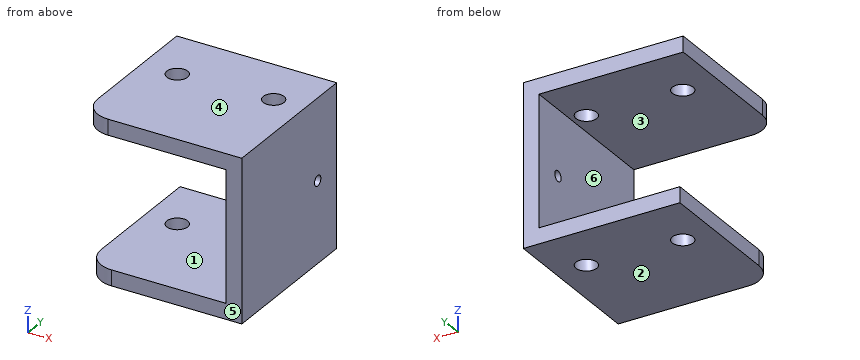
```python
from build123d import *

# Parameters (mm, degrees)
F1_DEPTH = 30
F3_D     = 2
F5_D     = 4
F6_R     = 5
F7_R     = 5


with BuildPart() as f1:
    # F0 (on Front) → F1 (new body)
    with BuildSketch(Plane.XZ):
        Polygon((-25.762998, -16.926608), (-25.762998, -19.926608), (4.237002, -19.926608), (4.237002, 11.073392), (-26.395301, 11.073392), (-26.395301, 8.073392), (1.237002, 8.073392), (1.237002, -16.926608), align=None)
    extrude(amount=F1_DEPTH)

    # F3 (through all)
    with Locations(Plane.YZ.offset(4.237002)):
        with Locations((-6, -4.426608)):
            Hole(F3_D / 2)

    # F5 (through all)
    with Locations(Plane(origin=(0, 0, -19.926608), x_dir=(1, 0, 0), z_dir=(0, 0, -1))):
        with Locations((-19.609278, 11.052052), (-1.659339, 10.208893)):
            Hole(F5_D / 2)

    # F6
    f6_edges = [f1.edges().sort_by_distance(p)[0] for p in [
        (-26.395301, -30, 9.573392),
    ]]
    fillet(f6_edges, radius=F6_R)

    # F7
    f7_edges = [f1.edges().sort_by_distance(p)[0] for p in [
        (-25.762998, -30, -18.426608),
    ]]
    fillet(f7_edges, radius=F7_R)


solid = f1.part
```
Verification items for the finished model (mm, model axes). Face numbers are marked on the shaded views. A direction names the side the tool comes from. Coordinates: 2 decimals unless noted, no trailing zeros. Loops run counter-clockwise (first coordinate to the right, second up) from the corner with the lowest first, then second, coordinate; pieces in that order, holes last. Notation, with made-up numbers: (32, 63) - (84, 63) arc R33 cw to (84, 100) - close; hole circle Ø2 at (48, 71.25). An arc over 180 degrees is marked (long way). Answer as a JSON object with one key per item and string values.
(1) Scan lines: line 1 along Z through (x, y) = (-9, -12); line 2 along Z through (x, y) = (3.15, -6); line 3 along X through (y, z) = (-24.5, 3). Record each from-to range of solid material in increasing order.
Response:
{"line 1": "z = -19.93 to -16.93, 8.07 to 11.07", "line 2": "z = -19.93 to -5.43, -3.43 to 11.07", "line 3": "x = 1.24 to 4.24"}
(2) Mould release check, pull along Z, two halves, no side actions. Record for the marked faces 3, 4, 5 and 6: pulls with the +Z half, pulls with the -Z half, needs draft (parallel to the pull), parting line crosses it, or undercut.
Response:
{"face 3": "undercut", "face 4": "pulls with the +Z half", "face 5": "needs draft", "face 6": "undercut"}
(3) Go/stop test with flat-tipped pins: pin 1 Ø3 at (x, y) = (-1.66, -10.21) entering from +Z; pin 2 Ø2.5 at (y, z) = (-7.5, -19) entering from -X; pin 3 Ø7.5 at (y, z) = (-9, -7.5) entering from -X. Record where each tip stops, or that it passes through.
Response:
{"pin 1": "passes through", "pin 2": "stops at x = -25.76", "pin 3": "stops at x = 1.24"}
(4) Cross-section at B-B, the plane y = -6. Record the boundary of the cut face in (x, z).
Response:
{"outline": "(-26.4, 8.07) - (1.24, 8.07) - (1.24, -3.43) - (4.24, -3.43) - (4.24, 11.07) - (-26.4, 11.07) - close; (-25.76, -19.93) - (4.24, -19.93) - (4.24, -5.43) - (1.24, -5.43) - (1.24, -16.93) - (-25.76, -16.93) - close"}
(5) Cross-section at A-A, the plane x = -4.5. Record the boundary of the cut face in (y, z).
Response:
{"outline": "(-30, -19.93) - (0, -19.93) - (0, -16.93) - (-30, -16.93) - close; (-30, 8.07) - (0, 8.07) - (0, 11.07) - (-30, 11.07) - close"}
(6) Access from +Z, -Z, +X, -X, +Y, -Y to the whole of each face (thin tool, end or side, straight path). Record for the marked faces 1 and 2.
Response:
{"face 1": "-X, +Y, -Y", "face 2": "-Z, +X, -X, +Y, -Y"}
(7) Cross-section at D-D, the plane x = -18.5. Record the boundary of the cut face in (y, z), then the cut area to 3 significant figures.
Response:
{"outline": "(-30, -19.93) - (-12.72, -19.93) - (-12.72, -16.93) - (-30, -16.93) - close; (-30, 8.07) - (-12.72, 8.07) - (-12.72, 11.07) - (-30, 11.07) - close; (-9.39, -19.93) - (0, -19.93) - (0, -16.93) - (-9.39, -16.93) - close; (-9.39, 8.07) - (0, 8.07) - (0, 11.07) - (-9.39, 11.07) - close", "area": "160 mm²"}
(8) Cross-section at C-C, the plane z = 8.5. Record the boundary of the cut face in (x, y).
Response:
{"outline": "(-26.4, -25) arc R5 ccw to (-21.4, -30) - (4.24, -30) - (4.24, 0) - (-26.4, 0) - close; hole circle Ø4 at (-19.61, -11.05); hole circle Ø4 at (-1.66, -10.21)"}
